Autodesk Inventor part; units mm, degrees
ref_plane "YZ Plane" through (0, 0, 0) normal (1, 0, 0) x (0, 1, 0)
ref_plane "XZ Plane" through (0, 0, 0) normal (0, 1, 0) x (-1, 0, 0)
ref_plane "XY Plane" through (0, 0, 0) normal (0, 0, 1) x (1, 0, 0)
sketch "스케치1" plane through (0, 0, 0) normal (1, 0, 0) x (0, 1, 0)
  line L0 (10.75, -9.25) -> (-10.75, -9.25)
  line L1 (-10.75, -9.25) -> (-10.75, 9.25)
  line L2 (-10.75, 9.25) -> (10.75, 9.25)
  line L3 (10.75, 9.25) -> (10.75, -9.25)
  line L4 (10.75, -9.25) -> (-10.75, 9.25) construction
  line L5 (-10.75, -9.25) -> (10.75, 9.25) construction
  line L6 (10.75, 7.75) -> (-9.25, 7.75)
  line L7 (-9.25, 7.75) -> (-9.25, 0.75)
  line L8 (-9.25, 0.75) -> (10.75, 0.75)
  line L9 (10.75, 0.75) -> (10.75, 7.75)
  line L10 (-9.25, -7.75) -> (10.75, -7.75)
  line L11 (-9.25, -0.75) -> (-9.25, -7.75)
  line L12 (10.75, -0.75) -> (-9.25, -0.75)
  line L13 (10.75, 9.25) -> (12.25, 9.25)
  line L14 (12.25, 9.25) -> (12.25, -9.25)
  line L15 (12.25, -9.25) -> (10.75, -9.25)
  line L16 (10.75, -9.25) -> (10.75, 9.25)
  point P0 (0, 0)
  point P1 (10.75, -7.75)
  point P2 (10.75, -0.75)
  point P3 (-10, 7.75)
  point P4 (-10, -7.75)
  point P5 (-10, 0.75)
  point P6 (-10, -0.75)
  point P7 (-10, -0.75)
  point P8 (-10, -7.75)
  dimension "d0" = 21.5
  dimension "d1" = 18.5
  dimension "d2" = 20
  dimension "d3" = 7
  dimension "d4" = 1.5
  dimension "d7" = 8.5
  dimension "d18" = 1.5
extrude "돌출1" add sketch "스케치1" against normal blind 45 contours L0 L1 L2 L3 L6 L7 L8 L12 L11 L10
sketch "스케치2" plane through (0, 0, 0) normal (1, 0, 0) x (0, 0, -1)
  line L0 (-9.25, -10.75) -> (9.25, -10.75)
  line L1 (-9.25, 10.75) -> (-9.25, -10.75)
  line L2 (-9.25, 10.75) -> (9.25, 10.75)
  line L3 (9.25, 10.75) -> (9.25, -10.75)
  line L4 (9.25, -10.75) -> (-9.25, -10.75)
  line L5 (-9.25, -10.75) -> (-9.25, 10.75)
  line L6 (9.25, 10.75) -> (-9.25, 10.75)
  line L7 (-9.25, 10.75) -> (-7.75, 10.75)
  point P0 (0, 0)
extrude "돌출2" add sketch "스케치2" along normal blind 1
sketch "스케치4" plane through (-45, -10.75, 9.25) normal (0, 0, 1) x (1, 0, 0)
  circle A0 centre (8.5, 19) radius 1.25
  circle A1 centre (26.5, 19) radius 1.25
  circle A2 centre (26.5, 4) radius 1.25
  circle A3 centre (8.5, 4) radius 1.25
  point P0 (45, 10.75)
extrude "돌출3" cut sketch "스케치4" against normal blind 45
sketch "스케치9" plane through (0, 10.75, 7.75) normal (0, 1, 0) x (1, 0, 0)
  line L0 (-45, 7) -> (-45, 8.5)
  line L1 (0, 7) -> (-45, 7)
  line L2 (-45, -1.5) -> (1, -1.5)
  line L3 (-45, 17) -> (1, 17)
  line L4 (-45, 17) -> (-35, 17)
  line L5 (-45, -1.5) -> (-35, -1.5)
  line L6 (-35, -1.5) -> (-35, -11.5)
  line L7 (-35, -11.5) -> (-45, -11.5)
  line L8 (-45, -11.5) -> (-45, -1.5)
  circle A0 centre (-40, -6.5) radius 2
  line L9 (-45, 7.75) -> (0, 7.75) construction
  line L10 (-22, -1.5) -> (-22, 17) construction
  line L11 (-35, 17) -> (-35, 27)
  line L12 (-35, 27) -> (-45, 27)
  line L13 (-45, 27) -> (-45, 17)
  circle A1 centre (-40, 22) radius 2
  line L14 (-45, 17) -> (-35, 17)
  line L15 (1, 17) -> (-9, 17)
  line L16 (1, -1.5) -> (-9, -1.5)
  line L17 (-9, -1.5) -> (-9, -11.5)
  line L18 (-9, -11.5) -> (1, -11.5)
  line L19 (1, -11.5) -> (1, -1.5)
  circle A2 centre (-4, -6.5) radius 2
  circle A3 centre (-4, 22) radius 2
  line L20 (-9, 17) -> (-9, 27)
  line L21 (-9, 27) -> (1, 27)
  line L22 (1, 27) -> (1, 17)
  line L23 (1, 17) -> (-9, 17)
  point P0 (-9, 17)
  dimension "d31" = 10
  dimension "d32" = 10
  dimension "d33" = 4
  dimension "d34" = 5
  dimension "d35" = 5
extrude "돌출6" add sketch "스케치9" against normal blind 1.5
sketch "스케치10" plane through (0, 0, 0) normal (-1, 0, 0) x (0, 0, 1)
  line L0 (-0.75, -9.25) -> (-0.75, 10.75)
  line L1 (-7.75, 10.75) -> (-0.75, 10.75)
  line L2 (-7.75, 10.75) -> (-7.75, -9.25)
  line L3 (-7.75, -9.25) -> (-0.75, -9.25)
  line L4 (1.75, 10.75) -> (1.75, -9.25)
  line L5 (1.75, -9.25) -> (7.75, -9.25)
  line L6 (7.75, 10.75) -> (7.75, -9.25)
  line L7 (1.75, 10.75) -> (7.75, 10.75)
  line L8 (0.75, 10.75) -> (0.75, -9.25)
  line L9 (0.75, -9.25) -> (7.75, -9.25)
  line L10 (7.75, -9.25) -> (7.75, 10.75)
  line L11 (0.75, 10.75) -> (7.75, 10.75)
  point P0 (0, 0)
extrude "돌출7" cut sketch "스케치10" against normal blind 10
properties part number "SAFRS-P-0031"
Here's how the part is built. I have some questions about the finished solid (model axes, mm). A direction names the side the tool comes from. Give positions to 0.01 mm unless a question says otherwise; leave off trailing zeros. Order: outer loops, then holes, each group sorted by start corner. A loop starts at its lowest first (then second) coordinate and runs counter-clockwise, first axis right, second up. Notation, with made-up numbers: M 88.5,-17 L 110.5,-17 A34 ccw 110.5,22 Z; hole C 47,-15 d11. An arc over 180 degrees is marked long. Use a Markdown table: item, result. Add a question column.
1. Suppose I cut it at B-B (z = -14.25). List the corners of the cut face in (x, y) for me, and give its area (3 significant figures).
2. I need wall thicknesses on probe 1 along Z at (x, y) = (-9, 9); probe 2 along Y at (x, z) = (-18.5, -0.2); probe 3 along X at (y, z) = (9.9, 14.25). Which ranges of each line are inside material? Lowest first, please. Write a range as from..to.
3. Suppose I cut it at C-C (y = 0). List the corners of the cut face in (x, z) for me.
4. Suppose I cut it at D-D (x = -29.5). List the corners of the cut face in (y, z) for me.
5. On a 3-axis mill with a long thin cutter (end or side, diameter ignored), from which of +Z, -Z, +X, -X, +Y, -Y can I reach the whole of each face in a straight line? I mean faces 5 (the flat face through (-4, 9.25, -12)), 6 (the cylindrical face through (-37.75, 8.3, 8.51)), 7 (the flat face through (-22, 1, 0.75)). Say none if no direction works.
6. Suppose I cut it at A-A (x = -4). List the corners of the cut face in (y, z) for me.
7. For pin 1 Ø10 at (x, y) = (-11.5, -1.5) entering from +Z; pin 2 Ø5 at (x, z) = (-4, -14.25) entering from -Y; pin 3 Ø8 at (y, z) = (-1.5, -2.5) entering from -X; pin 4 Ø6 at (x, y) = (-26, 3.5) entering from -Z, each with a flat end and sliding along its axis, tell me the tip position at first contact or that it passes through.
8. If we mould it in two halves opening along Y, with no side actions, what happens to faces 1 (the cylindrical face through (-37.75, 8.3, -8.49)), 2 (the flat face through (-35, 10, 14)), 3 (the flat face through (-37.8, 9.25, -14.3)), 4 (the cylindrical face through (-37.5, -7.5, 8.5))? For each: +Y half, -Y half, draft (parallel to the pull), parting line (faces both ways), or undercut.
Results list:
| question | item | result |
|---|---|---|
| 1 | outline | M -45,9.25 L -42,9.25 L -42,10.75 L -45,10.75 Z; M -38,9.25 L -35,9.25 L -35,10.75 L -38,10.75 Z; M -9,9.25 L -6,9.25 L -6,10.75 L -9,10.75 Z; M -2,9.25 L 1,9.25 L 1,10.75 L -2,10.75 Z |
| 1 | area | 18.0 mm² |
| 2 | probe 1 | z = -9.25..-7.75, -0.75..0.75, 7.75..9.25 |
| 2 | probe 2 | y = -10.75..-8, -5.5..7, 9.5..10.75 |
| 2 | probe 3 | x = -45..-42, -38..-35, -9..-6, -2..1 |
| 3 | outline | M -45,-9.25 L 1,-9.25 L 1,-7.75 L -45,-7.75 Z; M -45,-0.75 L 1,-0.75 L 1,0.75 L -45,0.75 Z; M -45,7.75 L 1,7.75 L 1,9.25 L -45,9.25 Z |
| 4 | outline | M -10.75,-9.25 L 10.75,-9.25 L 10.75,-7.75 L -9.25,-7.75 L -9.25,-0.75 L 10.75,-0.75 L 10.75,0.75 L -9.25,0.75 L -9.25,7.75 L 10.75,7.75 L 10.75,9.25 L -10.75,9.25 Z |
| 5 | face 5 | -Z, +X, -X, -Y |
| 5 | face 6 | none |
| 5 | face 7 | +X, -X, +Y |
| 6 | outline | M -10.75,-9.25 L 9.25,-9.25 L 9.25,-12.25 L 10.75,-12.25 L 10.75,-7.75 L -9.25,-7.75 L -9.25,-0.75 L 10.75,-0.75 L 10.75,0.75 L -9.25,0.75 L -9.25,7.75 L 10.75,7.75 L 10.75,12.25 L 9.25,12.25 L 9.25,9.25 L -10.75,9.25 Z; M 9.25,-19.25 L 10.75,-19.25 L 10.75,-16.25 L 9.25,-16.25 Z; M 9.25,16.25 L 10.75,16.25 L 10.75,19.25 L 9.25,19.25 Z |
| 7 | pin 1 | stops at z = 9.25 |
| 7 | pin 2 | stops at y = 9.25 |
| 7 | pin 3 | stops at x = -45 |
| 7 | pin 4 | stops at z = -9.25 |
| 8 | face 1 | undercut |
| 8 | face 2 | draft |
| 8 | face 3 | -Y half |
| 8 | face 4 | undercut |
